Source: three-view drawing plus pictorial views. Frame: mm from the lowest corner of the part. A direction names the side the tool comes from. Give positions to 0.01 mm unless a question says otherwise; leave off trailing zeros. Loops run counter-clockwise (first coordinate to the right, second up) from the corner with the lowest first, then second, coordinate; pieces in that order, holes last. Notation, with made-up numbers: M 61,81 L 114,81 A15 cw 114,96 Z; hole C 57.5,83 d11. An arc over 180 degrees is marked long. One line per item, written item: value. Start each with the question number.
(1) Pin query (flat end, axial travel): P1, Ø5, axis at x = 12, z = 31.5, coming from the -Y side; P2, Ø10, axis at y = 14.5, z = 13, coming from the +X side; P3, Ø15, axis at x = 47.5, y = 19, coming from the -Z side; P4, Ø4, axis at y = 8, z = 53, coming from the -X side. Return the tip coordinate at first contact, or that it passes through.
(2) Access query for the marked faces 1, 2 and 3. Directions: +Z, -Z, +X, -X, +Y, -Y. A direction counts if a zero-diameter tool reaches every point of the face in a straight line with its end or side. Return the directions, or none.
(3) Section A-A on y = 25. Output: boundary loops of the cut face in (x, z).
(4) Section D-D on z = 14.5. Output: boundary loops of the cut face in (x, y).
(5) Ray query, line 1 along Y through (x, z) = (12.5, 28); line 2 along X through (y, z) = (45.5, 64); line 3 along X through (y, z) = (10.5, 13.5). Return the intervals inside material, ascending. Write a range as from..to.
(6) Section C-C on z = 60. Output: boundary loops of the cut face in (x, y).
(7) Section B-B on x = 12.5. Output: boundary loops of the cut face in (y, z).
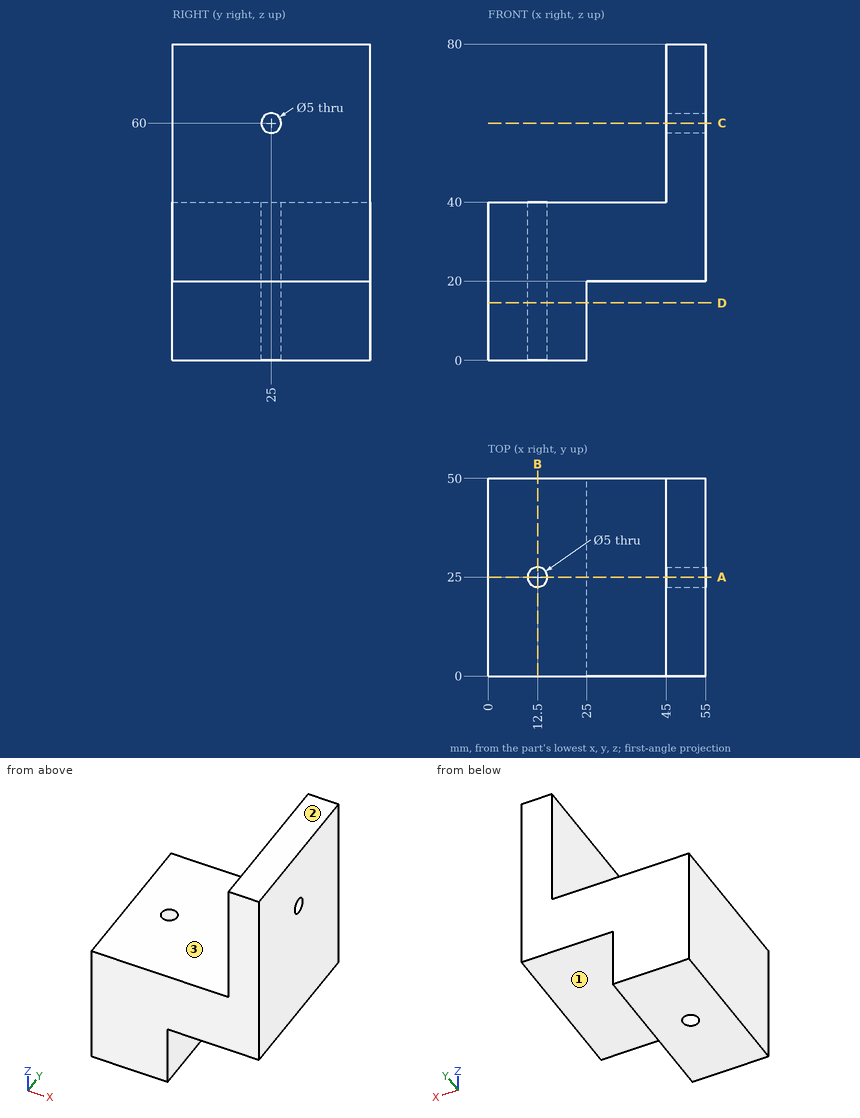
Output values:
1. P1: stops at y = 0
1. P2: stops at x = 25
1. P3: stops at z = 20
1. P4: stops at x = 45
2. face 1: -Z, +X, +Y, -Y
2. face 2: +Z, +X, -X, +Y, -Y
2. face 3: +Z, -X, +Y, -Y
3. outline: M 0,0 L 10,0 L 10,40 L 0,40 Z; M 15,0 L 25,0 L 25,20 L 55,20 L 55,57.5 L 45,57.5 L 45,40 L 15,40 Z; M 45,62.5 L 55,62.5 L 55,80 L 45,80 Z
4. outline: M 0,0 L 25,0 L 25,50 L 0,50 Z; hole C 12.5,25 d5
5. line 1: y = 0..22.5, 27.5..50
5. line 2: x = 45..55
5. line 3: x = 0..25
6. outline: M 45,0 L 55,0 L 55,22.5 L 45,22.5 Z; M 45,27.5 L 55,27.5 L 55,50 L 45,50 Z
7. outline: M 0,0 L 22.5,0 L 22.5,40 L 0,40 Z; M 27.5,0 L 50,0 L 50,40 L 27.5,40 Z
